Read the model definition and answer for the solid it produces. Units are mm, in the model's axes. A direction names the side the tool comes from. Coordinates: 2 decimals unless noted, no trailing zeros. Write each loop counter-clockwise with the first axis right and the second up, starting at its lowest first coordinate (ties: lowest second). Pieces come first, ordered by that corner, then holes.
from build123d import *

# Parameters (mm, degrees)
HOLE1_D           = 11.2268
HOLE1_DEPTH       = 33.3248
HOLE1_CSINK_D     = 12.7508
HOLE1_CSINK_ANGLE = 90


with BuildPart() as part:
    # Sketch1 → Revolve1 (revolve)
    with BuildSketch(Plane.XY):
        with BuildLine():
            Line((0, 0), (0, 8.58901))
            Line((0, 8.58901), (0.93599, 9.525))
            Line((0.93599, 9.525), (9.310047461, 9.525))
            Line((9.310047461, 9.525), (10.262333187, 8.610821042))
            ThreePointArc((10.262333187, 8.610821042), (10.619173954, 8.380210754), (11.0363, 8.29945))
            Line((11.0363, 8.29945), (12.3698, 8.29945))
            ThreePointArc((12.3698, 8.29945), (13.160062539, 8.626787461), (13.4874, 9.41705))
            Line((13.4874, 9.41705), (13.4874, 9.49325))
            Line((13.4874, 9.49325), (15.875, 9.49325))
            Line((15.875, 9.49325), (15.875, 0))
            Line((15.875, 0), (0, 0))
        make_face()
    revolve(axis=Axis((15.875, 0, 0), (-1, 0, 0)))

    # Sketch2 → Revolve2 (revolve)
    with BuildSketch(Plane.XY):
        Polygon((15.875, 0), (15.875, 19.76755), (20.6248, 19.76755), (20.6248, 18.18005), (21.6408, 18.18005), (22.6568, 19.19605), (26.2128, 19.19605), (26.9748, 18.43405), (26.9748, 0), align=None)
    revolve(axis=Axis((26.9748, 0, 0), (-1, 0, 0)))

    # Sketch3 → Revolve3 (revolve)
    with BuildSketch(Plane.XY):
        Polygon((26.9748, 0), (26.9748, 10.3124), (32.5628, 10.3124), (33.3248, 9.5504), (33.3248, 0), align=None)
    revolve(axis=Axis((33.3248, 0, 0), (-1, 0, 0)))

    # Hole1
    with Locations(Plane.ZY):
        with Locations((0, 0)):
            CounterSinkHole(HOLE1_D / 2, HOLE1_CSINK_D / 2, depth=HOLE1_DEPTH, counter_sink_angle=HOLE1_CSINK_ANGLE)

    # Sketch6 → Revolve4 (revolve)
    with BuildSketch(Plane.XY):
        with BuildLine():
            Line((20.6248, 17.92605), (21.6408, 17.92605))
            Line((21.6408, 17.92605), (21.6408, 18.18005))
            Line((21.6408, 18.18005), (21.1328, 18.18005))
            Line((21.1328, 18.18005), (20.758182072, 18.554667928))
            ThreePointArc((20.758182072, 18.554667928), (20.720984633, 18.64447049), (20.758182072, 18.734273051))
            Line((20.758182072, 18.734273051), (21.707290825, 19.683381804))
            Line((21.707290825, 19.683381804), (21.707290825, 19.76755))
            Line((21.707290825, 19.76755), (21.504090825, 19.76755))
            Line((21.504090825, 19.76755), (20.6248, 18.888259175))
            Line((20.6248, 18.888259175), (20.6248, 17.92605))
        make_face()
    revolve(axis=Axis((21.6408, 0, 0), (-1, 0, 0)))


solid = part.part
Item 1: Given pin 1 (2 mm diameter, centred on x = 21.5, y = -7, fed in from +Z); pin 2 (5 mm diameter, centred on x = 23.5, z = -3.5, fed in from +Y); pin 3 (2 mm diameter, centred on x = 21, z = 15.5, fed in from -Y); pin 4 (20 mm diameter, centred on y = 5, z = 4.5, fed in from -X), each flat-ended and moving along its own axis, determine where each tip first touches the part or whether it passes through.
Item 2: For faces 1 (the flat face through (26.975, 8, 8)), 2 (the cylindrical face through (17.27, -5.48, 1.22)), 3 (the cylindrical face through (11.7, -1.8, 8.1)), determine the directions among +Z, -Z, +X, -X, +Y, -Y from which every point of the face is accessible in a straight line to the end or side of a thin tool.
Item 3: Find the intervals of material crossed by probe 1 along Z at (x, y) = (19, 0); probe 2 along Z at (x, y) = (8, 0) (3 decimals); probe 3 along Y at (x, z) = (26, 0), in increasing order.
Item 4: The part is cut by section A-A (x = 31). Give the vertices of the cut face in (y, z).
Item 5: Determine the mould class of faces 4 (the flat face through (0, 1.3, -6.4)), 5 (the cylindrical face through (21.39, -3.94, 17.75)) for opening direction X: +X half, -X half, draft (parallel to the pull), parting line (faces both ways), or undercut.
Item 6: The part is cut by section B-B (x = 7.5). Give the vertices of the cut face in (y, z) (3 decimals), and give its area (3 significant figures).
Answer:
1. pin 1: stops at z = 18.83
1. pin 2: stops at y = 19.69
1. pin 3: stops at y = -13.36
1. pin 4: stops at x = 0
2. face 1: +X
2. face 2: +X, -X
2. face 3: none
3. probe 1: z = -19.77 to -5.61, 5.61 to 19.77
3. probe 2: z = -9.525 to -5.613, 5.613 to 9.525
3. probe 3: y = -19.2 to -5.61, 5.61 to 19.2
4. outline: circle Ø20.62 at (0, 0); hole circle Ø11.23 at (0, 0)
5. face 4: -X half
5. face 5: undercut
6. outline: circle Ø19.05 at (0, 0); hole circle Ø11.227 at (0, 0)
6. area: 186 mm2
